```python
from build123d import *

# Parameters (mm, degrees)
F0_R          = 19.05
F1_DEPTH      = 3.175
F3_DEPTH      = 3.175
F3_DEPTH_BACK = 3.175


with BuildPart() as f1:
    # F0 (on Front) → F1 (new body)
    with BuildSketch(Plane.XZ):
        Circle(F0_R)
    extrude(amount=F1_DEPTH)

    # F2 (on face) → F3 (join, two sides)
    with BuildSketch(Plane.XZ.offset(3.175)) as f3_sk:
        with BuildLine():
            Line((13.2951065898, 14.3205206841), (-11.1195538193, 14.3741192296))
            Line((-11.1195538193, 14.3741192296), (-10.3040672839, 13.5272685438))
            Line((-10.3040672839, 13.5272685438), (12.4042537063, 13.5272685438))
            Line((12.4042537063, 13.5272685438), (12.4042537063, 0.7942219963))
            add(Edge.make_bspline(
                [(12.4042537063, 0.7942219963), (12.2437335062, -0.6935312294), (11.9411104332, -3.4983399235), (10.9847031297, -5.6485725407), (10.5356024578, -6.6582583822)],
                knots=[0, 0, 0, 0, 0.5304294831, 1, 1, 1, 1], degree=3))
            Line((10.5356024578, -6.6582583822), (11.0988598317, -7.3030013591))
            add(Edge.make_bspline(
                [(11.0988598317, -7.3030013591), (11.6204761786, -6.0557843594), (12.6803886436, -3.521467994), (13.0880620978, -0.6713659701), (13.2951065898, 0.7761109737)],
                knots=[0, 0, 0, 0, 0.4921315337, 1, 1, 1, 1], degree=3))
            Line((13.2951065898, 0.7761109737), (13.2951065898, 14.3205206841))
        make_face()
        Polygon((-0.6866836248, -9.621998817), (-3.1270722393, -9.6166413277), (-1.1461181566, -11.1010298133), (-1.9328042399, -13.5020688176), (0.1275643008, -12.078541331), (2.1668851841, -13.4953176603), (1.4733931748, -11.1010298133), (3.3938813927, -9.6218636439), (0.9196144529, -9.6164317802), (0.0594901867, -7.3895342648), align=None)
        Polygon((9.7805182455, -10.2559360764), (11.5665001795, -10.2110812441), (11.5665001795, -8.3170095459), (5.9328516945, -2.6671725791), (4.9845642127, -3.6127429321), (11.1126137586, -9.7584016382), (9.7857490182, -9.7584016382), (4.7025149688, -4.7393189743), (4.6662185341, -5.2061798051), align=None)
        with BuildLine():
            Line((5.0151818607, -6.2073378134), (2.9217640404, -4.1403393261))
            add(Edge.make_bspline(
                [(2.9217640404, -4.1403393261), (4.0017596573, -3.2783505651), (6.2967614913, -1.4466155502), (6.3046824324, 4.5741096828), (0.6642850808, 8.0186176921), (-1.6742123718, 6.9825088021), (-2.6909445878, 6.5320292488)],
                knots=[0, 0, 0, 0, 0.2371028445, 0.503845992, 0.7842820981, 1, 1, 1, 1], degree=3))
            Line((-2.6909445878, 6.5320292488), (-9.8898978904, -0.6679674261))
            Line((-9.8898978904, -0.6679674261), (-8.5116093978, -0.6679674261))
            Line((-8.5116093978, -0.6679674261), (-6.13187678, 1.5893031363))
            Line((-6.13187678, 1.5893031363), (-2.3093123455, 1.5893031363))
            add(Edge.make_bspline(
                [(-2.3093123455, 1.5893031363), (-2.4412960331, 1.2516102423), (-2.7400240864, 0.4872859334), (-3.8346557693, 0.1745585357), (-4.445658531, 0)],
                knots=[0, 0, 0, 0, 0.441818859, 1, 1, 1, 1], degree=3))
            Line((-4.445658531, 0), (-6.857663393, 0))
            Line((-6.857663393, 0), (-11.7843858898, -4.9744602293))
            add(Edge.make_bspline(
                [(-11.7843858898, -4.9744602293), (-9.1052590566, -5.9842742459), (-4.2944262342, -7.7975689191), (-1.3186032332, -5.5161550663), (0, -4.5052482747)],
                knots=[0, 0, 0, 0, 0.5568946027, 1, 1, 1, 1], degree=3))
            add(Edge.make_bspline(
                [(0, -4.5052482747), (0.6645308371, -5.0850922819), (2.0325680841, -6.2787888796), (4.0022715592, -6.2316029467), (5.0151818607, -6.2073378134)],
                knots=[0, 0, 0, 0, 0.48575493, 1, 1, 1, 1], degree=3))
        make_face()
        with BuildLine():
            Line((9.138203226, -10.324401781), (8.6039779708, -9.8225530237))
            add(Edge.make_bspline(
                [(8.6039779708, -9.8225530237), (7.2581361134, -11.3018518624), (4.6817260383, -14.1337450832), (1.5133218063, -15.2414152892), (0, -15.7704707235)],
                knots=[0, 0, 0, 0, 0.5223709806, 1, 1, 1, 1], degree=3))
            add(Edge.make_bspline(
                [(-9.4586806372, -8.2151796669), (-8.2283692319, -9.8966299336), (-5.7644876665, -13.2639841641), (-1.9231894023, -14.9342388384), (0, -15.7704707235)],
                knots=[0, 0, 0, 0, 0.4993386949, 1, 1, 1, 1], degree=3))
            Line((-9.4586806372, -8.2151796669), (-10.7790241018, -8.2151796669))
            add(Edge.make_bspline(
                [(-10.7790241018, -8.2151796669), (-9.2866257772, -10.216307173), (-6.422821017, -14.1998498946), (-1.9977948837, -15.6756193291), (0, -16.4241865277)],
                knots=[0, 0, 0, 0, 0.5129628819, 1, 1, 1, 1], degree=3))
            add(Edge.make_bspline(
                [(9.138203226, -10.324401781), (7.6101712009, -11.8742374182), (5.1667983891, -14.7564398611), (1.7739776455, -15.8896886405), (0, -16.4241865277)],
                knots=[0, 0, 0, 0, 0.5144292418, 1, 1, 1, 1], degree=3))
        make_face()
        with BuildLine():
            Line((6.3793524168, -1.8924199976), (9.2547759414, -4.7678421251))
            add(Edge.make_bspline(
                [(-5.6524286047, 10.2112814784), (-3.6168299799, 11.2475901318), (0.8400975189, 13.5165799408), (10.0967712781, 7.8999192805), (11.6439949159, 0.4259003835), (10.018497176, -3.1076462689), (9.2547759414, -4.7678421251)],
                knots=[0, 0, 0, 0, 0.2433038431, 0.5327118892, 0.7804501082, 1, 1, 1, 1], degree=3))
            Line((-5.6524286047, 10.2112814784), (-2.9393755831, 7.4468469247))
            add(Edge.make_bspline(
                [(-2.9393755831, 7.4468469247), (-1.502485499, 7.851908623), (1.4748090248, 8.691212888), (6.2073016389, 5.7823119551), (7.5729609076, 0.7932677253), (6.7397473926, -1.0815105835), (6.3793524168, -1.8924199976)],
                knots=[0, 0, 0, 0, 0.255622974, 0.5296611682, 0.7965614469, 1, 1, 1, 1], degree=3))
        make_face()
        with BuildLine():
            Line((-3.3923503943, 6.5891323611), (-7.2932774201, 10.4900589213))
            add(Edge.make_bspline(
                [(-7.2932774201, 10.4900589213), (-7.0315208484, 10.6933025832), (-6.4937056941, 11.1108948549), (-5.835183803, 11.4424450599), (-5.4971668869, 11.6126285866)],
                knots=[0, 0, 0, 0, 0.4867035999, 1, 1, 1, 1], degree=3))
            Line((-5.4971668869, 11.6126285866), (-5.8058733121, 12.0335919783))
            add(Edge.make_bspline(
                [(-5.8058733121, 12.0335919783), (-6.6216145688, 11.4978026508), (-8.3538851706, 10.3600250858), (-9.8076282699, 8.3711164696), (-10.57679113, 7.3188021779)],
                knots=[0, 0, 0, 0, 0.4709086767, 1, 1, 1, 1], degree=3))
            Line((-10.57679113, 7.3188021779), (-10.1558286697, 6.9820312783))
            add(Edge.make_bspline(
                [(-8.1913326934, 9.5639401115), (-8.5656748556, 9.2353572907), (-9.3445869881, 8.5516588682), (-9.8785080222, 7.5186039785), (-10.1558286697, 6.9820312783)],
                knots=[0, 0, 0, 0, 0.4805961373, 1, 1, 1, 1], degree=3))
            Line((-8.1913326934, 9.5639401115), (-4.3044373822, 5.6770452643))
            Line((-4.3044373822, 5.6770452643), (-3.3923503943, 6.5891323611))
        make_face()
        Polygon((-5.0493629472, 4.9620792635), (-8.1632686779, 8.2449214533), (-8.1632686779, 7.6555726118), (-5.2445889451, 4.7649578191), align=None)
        with BuildLine():
            Line((-13.060814701, 13.2216596976), (-10.1942410693, 10.310985148))
            add(Edge.make_bspline(
                [(-10.1942410693, 10.310985148), (-10.4796394205, 9.9599556602), (-11.0312334616, 9.2815152529), (-11.4355277717, 8.6053887276), (-11.6306375712, 8.2790944725)],
                knots=[0, 0, 0, 0, 0.5174065165, 1, 1, 1, 1], degree=3))
            Line((-11.6306375712, 8.2790944725), (-11.0709676519, 7.8593418002))
            add(Edge.make_bspline(
                [(-11.0709676519, 7.8593418002), (-10.4892649761, 8.7107849431), (-9.2860247818, 10.4719778261), (-7.3393330178, 11.7938171812), (-6.3337632455, 12.4766174704)],
                knots=[0, 0, 0, 0, 0.4834468451, 1, 1, 1, 1], degree=3))
            Line((-6.3337632455, 12.4766174704), (-6.8334685639, 13.0362873897))
            add(Edge.make_bspline(
                [(-8.9322291315, 11.4572187886), (-8.6711328955, 11.7051084023), (-8.1063637602, 12.2413107045), (-7.2785688232, 12.7583035228), (-6.8334685639, 13.0362873897)],
                knots=[0, 0, 0, 0, 0.4623061346, 1, 1, 1, 1], degree=3))
            Line((-8.9322291315, 11.4572187886), (-11.8766472151, 14.3862600113))
            Line((-11.8766472151, 14.3862600113), (-11.5107083693, 14.935166575))
            Line((-11.5107083693, 14.935166575), (-11.8105309084, 15.1350488886))
            Line((-11.8105309084, 15.1350488886), (-12.5301061198, 15.1350488886))
            Line((-12.5301061198, 15.1350488886), (-12.7699645236, 14.935166575))
            add(Edge.make_bspline(
                [(-13.5973577846, 14.0257730544), (-13.7529213261, 14.2245779674), (-14.0633906595, 14.629918389), (-13.3650961838, 15.3086328914), (-12.9646191681, 15.0573192984), (-12.7699645236, 14.935166575)],
                knots=[0.0055616399, 0.0055616399, 0.0055616399, 0.0055616399, 0.3351525481, 0.6768462626, 1, 1, 1, 1], degree=3))
            Line((-13.5973577846, 14.0257730544), (-13.8105340302, 13.8158267364))
            Line((-13.8105340302, 13.8158267364), (-13.8105340302, 13.1114069372))
            Line((-13.8105340302, 13.1114069372), (-13.483288508, 12.8055869782))
            Line((-13.483288508, 12.8055869782), (-13.060814701, 13.2216596976))
        make_face()
        with BuildLine():
            Line((-13.1551567465, 12.3992469162), (-13.1551567465, 11.7663224228))
            Line((-13.1551567465, 11.7663224228), (-13.1551567465, 0))
            add(Edge.make_bspline(
                [(-11.9918715209, -4.4467356056), (-12.2321727364, -3.8322497133), (-12.7429395262, -2.5261431838), (-13.0124455989, -0.8745602441), (-13.1551567465, 0)],
                knots=[0, 0, 0, 0, 0.4704714955, 1, 1, 1, 1], degree=3))
            Line((-11.9918715209, -4.4467356056), (-11.3757159561, -3.8618131075))
            add(Edge.make_bspline(
                [(-11.3757159561, -3.8618131075), (-11.6411017383, -3.2356494914), (-12.168849425, -1.9904569373), (-12.1878234395, -0.6609463785), (-12.1972560883, 0)],
                knots=[0, 0, 0, 0, 0.5028648895, 1, 1, 1, 1], degree=3))
            Line((-12.1972560883, 0), (-12.5318219721, 11.7663224228))
            Line((-12.5318219721, 11.7663224228), (-13.1551567465, 12.3992469162))
        make_face()
    extrude(amount=F3_DEPTH)
    extrude(f3_sk.sketch, amount=-F3_DEPTH_BACK)


solid = f1.part
```
CAD build for the part. Positions are in the model's coordinates, mm. A direction names the side the tool comes from. Give positions to 0.01 mm unless a question says otherwise; leave off trailing zeros. Write each loop counter-clockwise with the first axis right and the second up, starting at its lowest first coordinate (ties: lowest second). Pieces come first, ordered by that corner, then holes. Notation, with made-up numbers: M -35.5,34 L -25.5,34 A13 cw -25.5,40 Z; hole C 21,-3.5 d8. An arc over 180 degrees is marked long. Return JSON: item names as keys, results as strings. Group by question number.
(1) Drill centre lines: L1, parallel to X at y = -4.75, z = 3; L2, parallel to X at y = -4.25, z = 0.5; L3, parallel to Z at x = -3.5, y = -4.5. Where is each one in solid material? Low to high. Write a range as [from, to].
(2) 3-axis set-ups, long thin cutter, end or side, ignore diameter. For faces 4 (the face through (7.797, -4.74, -3.31)), 5 (the face through (0, -6.35, -10)): which of +Z, -Z, +X, -X, +Y, -Y reach the whole face in a straight line?
(3) Band-saw the part on A-A (y = -5). State how many separate pieces and enclosed holes the cut face has, and give its area (3 significant figures).
(4) Mould opens along X. For faces 1 (the face through (-4.315, -4.74, 8.848)), 2 (the face through (13.295, -5, 7)), 3 (the face through (-6.73, -6.35, 6.51)) say: pulls with the +X half, pulls with the -X half, needs draft (parallel to the pull), parting line crosses it, or undercut.
(5) Flat gauge pins, fed straight in: pin 1 Ø1.2 at (x, y) = (-6, -5) entering from +Z; pin 2 Ø3.5 at (x, y) = (5.5, -5) entering from -Z; pin 3 Ø1 at (y, z) = (-5.5, 3) entering from -X. Where does each tip first touch, or does it go through?
(6) Band-saw the part on B-B (x = -16). Give the cut face in (y, z) (3 decimals).
Entries:
{
 "1": {"L1": "x = [-13.16, -12.28], [-6.22, 5.82], [6.83, 10.89], [12.4, 13.3]", "L2": "x = [-13.16, -12.21], [-8.72, -7.28], [-3.09, 6.07], [7.12, 10.98], [12.37, 13.26]", "L3": "z = [-15.04, -14.11], [-6.57, 0.3], [1.59, 5.72], [6.48, 6.7], [8.02, 11.24], [13.53, 14.36]"},
 "2": {"face 4": "-Y", "face 5": "+Z, -Z, +X, -X, -Y"},
 "3": {"separate pieces": "10", "enclosed holes": "0", "area": "370 mm^2"},
 "4": {"face 1": "undercut", "face 2": "pulls with the +X half", "face 3": "needs draft"},
 "5": {"pin 1": "stops at z = 14.36", "pin 2": "stops at z = -15.02", "pin 3": "stops at x = -13.16"},
 "6": {"outline": "M -3.175,-10.339 L 0,-10.339 L 0,10.339 L -3.175,10.339 Z"}
}
